Build history of the part. All positions in model axes, mm. A direction names the side the tool comes from. Give positions to 0.01 mm unless a question says otherwise; leave off trailing zeros. Write each loop counter-clockwise with the first axis right and the second up, starting at its lowest first coordinate (ties: lowest second). Pieces come first, ordered by that corner, then holes. Notation, with made-up numbers: (-0.75, 38.5) -> (47.25, 38.5) arc R25 ccw to (47.25, 64.5) -> close; hole circle Ø2 at (78.25, -33.75). An arc over 180 degrees is marked (long way). Put each result on its own line as item: value.
from build123d import *

# Parameters (mm, degrees)
SKETCH_R        = 1.55
SKETCH_W        = 6.5
SKETCH_H        = 3
SKETCH_W_2      = 11.5
PAD_DEPTH       = 5.4
SKETCH005_W     = 25.7
SKETCH005_H     = 13
POCKET_DEPTH    = 3
SKETCH006_R     = 1.8
POCKET001_DEPTH = 1.4
POCKET002_DEPTH = 3
FILLET_R        = 1
FILLET001_R     = 0.5


with BuildPart() as part:
    # Sketch → Pad (new body)
    with BuildSketch(Plane.XY):
        with BuildLine():
            Line((-2, 13.5), (2, 13.5))
            ThreePointArc((15.5, 0), (11.545942, 9.545942), (2, 13.5))
            Line((15.5, 0), (15.5, -25.7))
            ThreePointArc((12.7, -28.5), (14.679899, -27.679899), (15.5, -25.7))
            Line((11, -28.5), (12.7, -28.5))
            Line((11, -29.7), (11, -28.5))
            Line((-3, -29.7), (11, -29.7))
            Line((-3, -31.15), (-3, -29.7))
            Line((-3, -31.15), (-15.5, -31.15))
            Line((-15.5, -31.15), (-15.5, 0))
            ThreePointArc((-2, 13.5), (-11.545942, 9.545942), (-15.5, 0))
        make_face()
        with Locations((-11, -11)):
            Circle(SKETCH_R, mode=Mode.SUBTRACT)
        with Locations((11, -11)):
            Circle(SKETCH_R, mode=Mode.SUBTRACT)
        with BuildLine():
            ThreePointArc((-3.919184, 9.2), (-10, 0), (-3.919184, -9.2))
            Line((3.919184, -9.2), (-3.919184, -9.2))
            ThreePointArc((3.919184, -9.2), (10, 0), (3.919184, 9.2))
            Line((-3.919184, 9.2), (3.919184, 9.2))
        make_face(mode=Mode.SUBTRACT)
        with Locations((-8.91, -25.81)):
            Rectangle(SKETCH_W, SKETCH_H, mode=Mode.SUBTRACT)
        with Locations((6.35, -25.81)):
            Rectangle(SKETCH_W_2, SKETCH_H, mode=Mode.SUBTRACT)
    extrude(amount=PAD_DEPTH)

    # Sketch005 (on Face26 of Pad) → Pocket (cut)
    with BuildSketch(Plane(origin=(0, 0, 0), x_dir=(1, 0, 0), z_dir=(0, 0, -1))):
        with Locations((0, 22)):
            Rectangle(SKETCH005_W, SKETCH005_H)
    extrude(amount=-POCKET_DEPTH, mode=Mode.SUBTRACT)

    # Sketch006 (on Face32 of Pocket) → Pocket001 (cut)
    with BuildSketch(Plane(origin=(0, 0, 3), x_dir=(1, 0, 0), z_dir=(0, 0, -1))):
        with Locations((0, 22)):
            Circle(SKETCH006_R)
        with BuildLine():
            Line((-12.85, 20.5), (-3.5, 20.5))
            ThreePointArc((-1.5, 18.5), (-2.085786, 19.914214), (-3.5, 20.5))
            Line((-1.5, 18.5), (-1.5, 15.5))
            Line((-1.5, 15.5), (-12.85, 15.5))
            Line((-12.85, 15.5), (-12.85, 20.5))
        make_face()
        with BuildLine():
            Line((1.5, 15.5), (12.85, 15.5))
            Line((12.85, 15.5), (12.85, 20.5))
            Line((12.85, 20.5), (3.5, 20.5))
            ThreePointArc((3.5, 20.5), (2.085786, 19.914214), (1.5, 18.5))
            Line((1.5, 18.5), (1.5, 15.5))
        make_face()
        with BuildLine():
            Line((-12.85, 23.5), (-3.5, 23.5))
            ThreePointArc((-3.5, 23.5), (-2.085786, 24.085786), (-1.5, 25.5))
            Line((-1.5, 25.5), (-1.5, 28.5))
            Line((-1.5, 28.5), (-12.85, 28.5))
            Line((-12.85, 28.5), (-12.85, 23.5))
        make_face()
        with BuildLine():
            Line((1.5, 28.5), (12.85, 28.5))
            Line((12.85, 28.5), (12.85, 23.5))
            Line((12.85, 23.5), (3.5, 23.5))
            ThreePointArc((1.5, 25.5), (2.085786, 24.085786), (3.5, 23.5))
            Line((1.5, 25.5), (1.5, 28.5))
        make_face()
    extrude(amount=-POCKET001_DEPTH, mode=Mode.SUBTRACT)

    # Sketch001 (on Face5 of Pocket001) → Pocket002 (cut)
    with BuildSketch(Plane.XY.offset(5.4)):
        Polygon((-8, -12.732051), (-8, -9.267949), (-11, -7.535898), (-14, -9.267949), (-14, -12.732051), (-11, -14.464102), align=None)
        Polygon((14, -12.732051), (14, -9.267949), (11, -7.535898), (8, -9.267949), (8, -12.732051), (11, -14.464102), align=None)
    extrude(amount=-POCKET002_DEPTH, mode=Mode.SUBTRACT)

    # Fillet
    fillet_edges = [part.edges().sort_by_distance(p)[0] for p in [
        (-15.5, -31.15, 2.7),
        (-3, -31.15, 2.7),
        (11, -29.7, 2.7),
    ]]
    fillet(fillet_edges, radius=FILLET_R)

    # Fillet001
    fillet001_edges = [part.edges().sort_by_distance(p)[0] for p in [
        (12.85, -23.5, 3.7),
        (12.85, -20.5, 3.7),
        (-12.85, -20.5, 3.7),
        (-12.85, -23.5, 3.7),
        (-1.8, -22, 4.4),
        (0.6, -27.31, 4.2),
        (0.6, -24.31, 4.2),
        (1.892549, -24.31, 3.7),
        (-3, -29.7, 2.7),
        (12.1, -27.31, 4.9),
        (12.1, -24.31, 4.9),
        (-5.66, -27.31, 4.9),
        (-5.66, -24.31, 4.9),
        (-12.16, -24.31, 4.9),
        (-12.16, -27.31, 4.9),
        (-12.85, -15.5, 1.5),
        (12.85, -28.495979, 1.5),
        (9.45, -11, 0),
        (-12.55, -11, 0),
    ]]
    fillet(fillet001_edges, radius=FILLET001_R)


solid = part.part
1) Slice it at B-B (y = -3.5). Write the cut outline in (x, z).
Filled sheet:
outline: (-15.5, 0) -> (-9.37, 0) -> (-9.37, 5.4) -> (-15.5, 5.4) -> close; (9.37, 0) -> (15.5, 0) -> (15.5, 5.4) -> (9.37, 5.4) -> close
2) Tool access for faces 1 (the flat face through (12, -28.5, 5)), 2 (the flat face through (0, -15.5, 2)), 3 (the flat face through (12.5, -13.6, 3.9)), 4 (the flat face through (6, -27.31, 5)): list every direction of +Z, -Z, +X, -X, +Y, -Y with a clear straight run to the whole face (end or side of a thin tool).
Filled sheet:
face 1: +Z, -Z, +X, -Y
face 2: -Z
face 3: +Z
face 4: +Z, -Z
3) Slice it at D-D (z = 1.7). Give the number of separate pieces and of enclosed holes in the cut face, plus the area to 3 significant figures.
Filled sheet:
separate pieces: 1
enclosed holes: 3
area: 616 mm2
4) Wall check: L1, parallel to X at y = -11, z = 1.25; L2, parallel to X at y = -20.5, z = 0.3; L3, parallel to Y at x = -11, z = 0.9. Give the ranges that are in metal, low to high.
Filled sheet:
L1: -15.5 to -12.55, -9.45 to 9.45, 12.55 to 15.5
L2: -15.5 to -12.85, 12.85 to 15.5
L3: -31.15 to -28.5, -15.5 to -12.55, -9.45 to 10.06
5) Slice it at A-A (x = 0). Write the cut outline in (y, z), plus the area to 3 significant figures.
Filled sheet:
outline: (-29.7, 0) -> (-28.5, 0) -> (-28.5, 3) -> (-23.8, 3) -> (-23.8, 3.9) arc R0.5 cw to (-23.3, 4.4) -> (-20.7, 4.4) arc R0.5 cw to (-20.2, 3.9) -> (-20.2, 3) -> (-15.5, 3) -> (-15.5, 0) -> (-9.2, 0) -> (-9.2, 5.4) -> (-29.7, 5.4) -> close; (9.2, 0) -> (13.5, 0) -> (13.5, 5.4) -> (9.2, 5.4) -> close
area: 90.0 mm2
6) Pull direction X, two halves, no side cores. Call faces 5 (the flat face through (0, 13.5, 3)), 6 (the cylindrical face through (15, -27.3, 2.7)), 7 (the flat face through (-1.5, -17, 4)): released by +X, released by -X, zero draft, split by the parting line, or undercut.
Filled sheet:
face 5: zero draft
face 6: released by +X
face 7: undercut
7) Pin check, flat tips, straight feed: pin 1 (2 mm diameter, centred on x = 6.5, z = 1.5, fed in from -Y); pin 2 (1.5 mm diameter, centred on x = -7, z = 3.5, fed in from +Y); pin 3 (1.8 mm diameter, centred on x = -10, y = -11.5, fed in from +Z). Stop position of each tip, or through.
Filled sheet:
pin 1: y = -29.7
pin 2: y = 12.81
pin 3: z = 2.4
8) Slice it at C-C (x = -7). Write the cut outline in (y, z), plus the area to 3 significant figures.
Filled sheet:
outline: (-31.15, 0) -> (-28.5, 0) -> (-28.5, 4.4) -> (-27.31, 4.4) -> (-27.31, 5.4) -> (-31.15, 5.4) -> close; (-24.31, 4.4) -> (-23.5, 4.4) -> (-23.5, 3) -> (-20.5, 3) -> (-20.5, 4.4) -> (-15.5, 4.4) -> (-15.5, 0) -> (-7.14, 0) -> (-7.14, 5.4) -> (-24.31, 5.4) -> close; (7.14, 0) -> (12.54, 0) -> (12.54, 5.4) -> (7.14, 5.4) -> close
area: 103 mm2
